Design review of the part built by this model. Coordinates are the model's own, in mm. Round coordinates to 2 decimals unless told otherwise and drop trailing zeros. Loops run counter-clockwise (first coordinate to the right, second up) from the corner with the lowest first, then second, coordinate; pieces in that order, holes last. Notation, with made-up numbers: (2.25, 83.5) -> (42.25, 83.5) arc R24 ccw to (42.25, 101.5) -> close; hole circle Ø4 at (-29, 83). An arc over 180 degrees is marked (long way). Answer as CSV lines item,"result". Start each with the question number.
(1) For P1, Ø12, axis at x = -14, z = -139.5, coming from the +Y side; P2, Ø13, axis at x = -0.5, y = 172, coming from the -Z side, all flat-tipped, find the tip position at first contact; note any pin that passes through.
(2) Draft analysis for pull direction Z (two halves, no side actions). For faces 1 (the face through (0, 0, -131)), 2 (the face through (0, 127, -110)), 3 (the face through (-12.84, -0.608, -133.356)), state which applies: +Z half, -Z half, draft (parallel to the pull), parting line (faces both ways), or undercut.
(3) Take a section at A-A, the plane y = 72.8. Write out the cut boundary in (x, z).
(4) Take a section at D-D, the plane y = 165.5. Write out the cut boundary in (x, z), and give its area (3 significant figures).
(5) Take a section at B-B, the plane x = 0. Write out the cut boundary in (y, z).
(6) Take a section at C-C, the plane x = 18.5. Write out the cut boundary in (y, z).
(7) To check wall thickness, follow line 1 (Y direction, x = 5, z = -126); line 2 (Z direction, x = 3.5, y = 210.5). State the ranges of each line that lie inside material, in increasing order. Write a range as from..to.
from build123d import *

# Parameters (mm, degrees)
SKETCH1_W              = 44
SKETCH1_H              = 300
BASE_FLANGE1_DEPTH     = 1.2
SKETCHED_START         = -22
SKETCHED_BEND1_DEPTH   = 44
SKETCHED_BEND1_2_DEPTH = 44
SKETCH7_R              = 4
CUT_EXTRUDE1_DEPTH     = 10
SKETCH9_R              = 3.234304459
CUT_EXTRUDE2_DEPTH     = 10


# Read off the part's stored shape, not the designer's step: Sketched Bend1
# Sheet-metal steps are written as plain solids
with BuildPart() as part:
    # Sketch1 → Base-Flange1 (new body)
    with BuildSketch(Plane(origin=(0, 0, 0), x_dir=(1, 0, 0), z_dir=(0, 1, 0))):
        Rectangle(SKETCH1_W, SKETCH1_H)
    extrude(amount=-BASE_FLANGE1_DEPTH)

    # Sketched Bend1 outline → Sketched Bend1 (cut)
    with BuildSketch(Plane.YZ.offset(SKETCHED_START)):
        with BuildLine():
            ThreePointArc((-1.2, -110.7366), (-0.872269031, -109.658657516), (0, -108.945555612))
            Line((0, -108.945555612), (0, 150))
            Line((0, 150), (-1.2, 150))
            Line((-1.2, 150), (-1.2, -110.7366))
        make_face()
    extrude(amount=SKETCHED_BEND1_DEPTH, mode=Mode.SUBTRACT)

    # Sketched Bend1 2 outline → Sketched Bend1 2 (add)
    with BuildSketch(Plane.YZ.offset(SKETCHED_START)):
        with BuildLine():
            Line((257.6, -110), (257.6, -108.8))
            Line((257.6, -108.8), (0.7366, -108.8))
            ThreePointArc((0.7366, -108.8), (0.361178238, -108.836737358), (0, -108.945555612))
            Line((0, -108.945555612), (0, -110.7366))
            ThreePointArc((0, -110.7366), (0.215745145, -110.215745145), (0.7366, -110))
            Line((0.7366, -110), (257.6, -110))
        make_face()
    extrude(amount=SKETCHED_BEND1_2_DEPTH)

    # Sketch7 → Cut-Extrude1 (cut)
    with BuildSketch(Plane.XY.offset(-108.8)):
        with Locations((0, 72.8)):
            Circle(SKETCH7_R)
        with Locations((0, 212.8)):
            Circle(SKETCH7_R)
    extrude(amount=-CUT_EXTRUDE1_DEPTH, mode=Mode.SUBTRACT)

    # Sketch9 → Cut-Extrude2 (cut)
    with BuildSketch(Plane.XZ.offset(1.2)):
        with Locations(Location((-11.601340887, -130.3683, 0), (0, 0, 270))):
            Circle(SKETCH9_R)
        with Locations(Location((11.601340887, -130.3683, 0), (0, 0, 270))):
            Circle(SKETCH9_R)
    extrude(amount=-CUT_EXTRUDE2_DEPTH, mode=Mode.SUBTRACT)


solid = part.part
The answers:
1,P1,"y = 0"
1,P2,"z = -110"
2,face 1,"draft"
2,face 2,"-Z half"
2,face 3,"undercut"
3,outline,"(-22, -110) -> (-4, -110) -> (-4, -108.8) -> (-22, -108.8) -> close; (4, -110) -> (22, -110) -> (22, -108.8) -> (4, -108.8) -> close"
4,outline,"(-22, -110) -> (22, -110) -> (22, -108.8) -> (-22, -108.8) -> close"
4,area,"52.8 mm²"
5,outline,"(-1.2, -150) -> (0, -150) -> (0, -110.74) arc R0.74 cw to (0.74, -110) -> (68.8, -110) -> (68.8, -108.8) -> (0.74, -108.8) arc R1.94 ccw to (-1.2, -110.74) -> close; (76.8, -110) -> (208.8, -110) -> (208.8, -108.8) -> (76.8, -108.8) -> close; (216.8, -110) -> (257.6, -110) -> (257.6, -108.8) -> (216.8, -108.8) -> close"
6,outline,"(-1.2, -150) -> (0, -150) -> (0, -110.74) arc R0.74 cw to (0.74, -110) -> (257.6, -110) -> (257.6, -108.8) -> (0.74, -108.8) arc R1.94 ccw to (-1.2, -110.74) -> close"
7,line 1,"-1.2..0"
7,line 2,"-110..-108.8"
